```python
from build123d import *

# Parameters (mm, degrees)
BOSS_EXTRUDE1_DEPTH                 = 12.5
CUT_EXTRUDE1_REACH                  = 42.463
CUT_EXTRUDE1_END_RADIUS             = 9.5
CUT_EXTRUDE1_DIRECTION_2_REACH      = 42.463
CUT_EXTRUDE1_DIRECTION_2_END_RADIUS = 9.5
BOSS_EXTRUDE3_DEPTH                 = 6.35
SKETCH5_R                           = 2.5
BOSS_EXTRUDE4_DEPTH                 = 6.35
BOSS_EXTRUDE5_START                 = -46
BOSS_EXTRUDE5_DEPTH                 = 46
BOSS_EXTRUDE6_DEPTH                 = 6.35
BOSS_EXTRUDE6_DRAFT                 = 10
HOLE1_START                         = 6.15
HOLE1_OUTLINE_R                     = 2.5
HOLE1_DEPTH                         = 52.35
FILLET1_R                           = 2.5


# Read off the part's stored shape, not the designer's step: Hole1
with BuildPart() as part:
    # Sketch1 → Boss-Extrude1 (new, symmetric)
    with BuildSketch(Plane.XY):
        with BuildLine():
            ThreePointArc((-9.5, 12.87439319), (-35, 0), (-9.5, -12.87439319))
            ThreePointArc((-9.5, -12.87439319), (0, -9.748786379), (9.5, -12.87439319))
            ThreePointArc((9.5, -12.87439319), (35, 0), (9.5, 12.87439319))
            ThreePointArc((9.5, 12.87439319), (0, 9.748786379), (-9.5, 12.87439319))
        make_face()
    extrude(amount=BOSS_EXTRUDE1_DEPTH, both=True)

    # Sketch2 → Cut-Revolve1 (revolve, cut)
    with BuildSketch(Plane(origin=(19, 0, 0), x_dir=(0, 0, -1), z_dir=(1, 0, 0)), mode=Mode.PRIVATE) as cut_revolve1_sk:
        Polygon((-12.5, 0), (-12.5, 14.25), (-6.5, 14.25), (-6.5, 12.5), (-4.5, 12.5), (-4.5, 11.5), (-2.5, 11.5), (-2.5, 9.5), (9.5, 9.5), (9.5, 4.5), (8.5, 4.5), (8.5, 0), align=None)
    cut_revolve1 = revolve(cut_revolve1_sk.sketch.rotate(Axis((19, 0, 0), (0, 0, 1)), 90), axis=Axis((19, 0, 0), (0, 0, 1)), mode=Mode.SUBTRACT)

    # Mirror1: Cut-Revolve1 across plane
    add(cut_revolve1.mirror(Plane(origin=(0, 0, 0), x_dir=(0, 0, 1), z_dir=(1, 0, 0))), mode=Mode.SUBTRACT)

    # Cut-Extrude1: up to this cylinder (the profile starts outside it)
    cut_extrude1_end = Plane(origin=(-19, 0, 0), z_dir=(0, 0, -1)) * Cylinder(CUT_EXTRUDE1_END_RADIUS, 104.926, mode=Mode.PRIVATE)
    # Sketch3 → Cut-Extrude1 (cut, up to the surface)
    with BuildSketch(Plane(origin=(0, 0, 0), x_dir=(0, 0, -1), z_dir=(1, 0, 0)), mode=Mode.PRIVATE) as cut_extrude1_sk1:
        with BuildLine():
            Line((0.75, -7.75), (-0.75, -7.75))
            ThreePointArc((-0.75, -7.75), (-1.810660172, -7.310660172), (-2.25, -6.25))
            Line((-2.25, -6.25), (-2.25, 6.25))
            ThreePointArc((-2.25, 6.25), (-1.810660172, 7.310660172), (-0.75, 7.75))
            Line((-0.75, 7.75), (0.75, 7.75))
            ThreePointArc((0.75, 7.75), (1.810660172, 7.310660172), (2.25, 6.25))
            Line((2.25, 6.25), (2.25, -6.25))
            ThreePointArc((2.25, -6.25), (1.810660172, -7.310660172), (0.75, -7.75))
        make_face()
    cut_extrude1_tool1 = extrude(cut_extrude1_sk1.sketch, amount=-CUT_EXTRUDE1_REACH, mode=Mode.PRIVATE) - cut_extrude1_end
    add(cut_extrude1_tool1.solids().sort_by_distance((0, 0, 0))[0], mode=Mode.SUBTRACT)

    # Cut-Extrude1 direction 2: up to this cylinder (the profile starts outside it)
    cut_extrude1_direction_2_end = Plane(origin=(19, 0, 0), z_dir=(0, 0, -1)) * Cylinder(CUT_EXTRUDE1_DIRECTION_2_END_RADIUS, 104.926, mode=Mode.PRIVATE)
    # Sketch3 → Cut-Extrude1 direction 2 (cut, up to the surface)
    with BuildSketch(Plane(origin=(0, 0, 0), x_dir=(0, 0, -1), z_dir=(1, 0, 0)), mode=Mode.PRIVATE) as cut_extrude1_direction_2_sk1:
        with BuildLine():
            Line((0.75, -7.75), (-0.75, -7.75))
            ThreePointArc((-0.75, -7.75), (-1.810660172, -7.310660172), (-2.25, -6.25))
            Line((-2.25, -6.25), (-2.25, 6.25))
            ThreePointArc((-2.25, 6.25), (-1.810660172, 7.310660172), (-0.75, 7.75))
            Line((-0.75, 7.75), (0.75, 7.75))
            ThreePointArc((0.75, 7.75), (1.810660172, 7.310660172), (2.25, 6.25))
            Line((2.25, 6.25), (2.25, -6.25))
            ThreePointArc((2.25, -6.25), (1.810660172, -7.310660172), (0.75, -7.75))
        make_face()
    cut_extrude1_direction_2_tool1 = extrude(cut_extrude1_direction_2_sk1.sketch, amount=CUT_EXTRUDE1_DIRECTION_2_REACH, mode=Mode.PRIVATE) - cut_extrude1_direction_2_end
    add(cut_extrude1_direction_2_tool1.solids().sort_by_distance((0, 0, 0))[0], mode=Mode.SUBTRACT)

    # Sketch4 → Boss-Extrude3 (add)
    with BuildSketch(Plane.XY.offset(12.5)):
        with BuildLine():
            Line((-45.380476721, -5.413087491), (-34.979470203, -0.810266645))
            ThreePointArc((-34.979470203, -0.810266645), (-31.820655502, -9.572397426), (-24.317188777, -15.090642912))
            Line((-24.317188777, -15.090642912), (-44.730811053, -13.974760557))
            ThreePointArc((-44.730811053, -13.974760557), (-47.485667167, -9.87831587), (-45.380476721, -5.413087491))
        make_face()
    boss_extrude3 = extrude(amount=-BOSS_EXTRUDE3_DEPTH)

    # Mirror2: Boss-Extrude3 across plane
    add(boss_extrude3.mirror(Plane(origin=(0, 0, 0), x_dir=(0, 0, 1), z_dir=(1, 0, 0))))

    # Sketch5 → Boss-Extrude4 (add)
    with BuildSketch(Plane.XY.offset(12.5)):
        with BuildLine():
            ThreePointArc((-14.279554898, 31.478453226), (-19, 34.83), (-23.720445102, 31.478453226))
            Line((-23.720445102, 31.478453226), (-31.028962191, 10.550074342))
            ThreePointArc((-31.028962191, 10.550074342), (-20.717418693, 15.907560248), (-9.5, 12.87439319))
            ThreePointArc((-9.5, 12.87439319), (-8.431487389, 12.150623988), (-7.308118696, 11.515325762))
            Line((-7.308118696, 11.515325762), (-14.279554898, 31.478453226))
        make_face()
        with Locations((-19, 29.83)):
            Circle(SKETCH5_R, mode=Mode.SUBTRACT)
    extrude(amount=-BOSS_EXTRUDE4_DEPTH)

    # Sketch6 → Boss-Extrude5 (add)
    with BuildSketch(Plane(origin=(0, 0, 6.15), x_dir=(-1, 0, 0), z_dir=(0, 0, -1)).offset(BOSS_EXTRUDE5_START)):
        with BuildLine():
            Line((44.730811053, -13.974760557), (24.317188777, -15.090642912))
            ThreePointArc((24.317188777, -15.090642912), (16.633162841, -15.823971747), (9.5, -12.87439319))
            ThreePointArc((9.5, -12.87439319), (0, -9.748786379), (-9.5, -12.87439319))
            ThreePointArc((-9.5, -12.87439319), (-16.633162841, -15.823971747), (-24.317188777, -15.090642912))
            Line((-24.317188777, -15.090642912), (-44.730811053, -13.974760557))
            ThreePointArc((-44.730811053, -13.974760557), (0, -32.403655151), (44.730811053, -13.974760557))
        make_face()
    extrude(amount=BOSS_EXTRUDE5_DEPTH)


with BuildPart() as boss_extrude6_tool:
    # Sketch7 → Boss-Extrude6 (with draft: the straight prism first)
    with BuildSketch(Plane.XY.offset(52.15)):
        with BuildLine():
            Line((-7.5, 15.5), (-7.5, 9.15))
            ThreePointArc((-7.5, 9.15), (-19, -2.35), (-30.5, 9.15))
            Line((-30.5, 9.15), (-30.5, 15.5))
            Line((-30.5, 15.5), (-40, 15.5))
            Line((-40, 15.5), (-40, 8.234972412))
            ThreePointArc((-40, 8.234972412), (-41.393677612, 0.899799121), (-45.380476721, -5.413087491))
            ThreePointArc((-45.380476721, -5.413087491), (-47.485667167, -9.87831587), (-44.730811053, -13.974760557))
            ThreePointArc((-44.730811053, -13.974760557), (0, -32.403655151), (44.730811053, -13.974760557))
            ThreePointArc((44.730811053, -13.974760557), (47.485667167, -9.87831587), (45.380476721, -5.413087491))
            ThreePointArc((45.380476721, -5.413087491), (41.393677612, 0.899799121), (40, 8.234972412))
            Line((40, 8.234972412), (40, 15.5))
            Line((40, 15.5), (30.5, 15.5))
            Line((30.5, 15.5), (30.5, 9.15))
            ThreePointArc((30.5, 9.15), (19, -2.35), (7.5, 9.15))
            Line((7.5, 9.15), (7.5, 15.5))
            Line((7.5, 15.5), (-7.5, 15.5))
        make_face()
    extrude(amount=BOSS_EXTRUDE6_DEPTH)
    # Boss-Extrude6: the draft: its side faces are tilted about the plane it starts from
    boss_extrude6_sides = [boss_extrude6_tool.faces().sort_by_distance(p)[0] for p in [
        (0, -32.403655151, 55.325),
        (47.485667167, -9.87831587, 55.325),
        (41.393677612, 0.899799121, 55.325),
        (40, 11.867486206, 55.325),
        (35.25, 15.5, 55.325),
        (30.5, 12.325, 55.325),
        (19, -2.35, 55.325),
        (7.5, 12.325, 55.325),
        (0, 15.5, 55.325),
        (-7.5, 12.325, 55.325),
        (-19, -2.35, 55.325),
        (-30.5, 12.325, 55.325),
        (-35.25, 15.5, 55.325),
        (-40, 11.867486206, 55.325),
        (-41.393677612, 0.899799121, 55.325),
        (-47.485667167, -9.87831587, 55.325),
    ]]
    draft(boss_extrude6_sides, Plane.XY.offset(52.15), BOSS_EXTRUDE6_DRAFT)


with BuildPart() as part_1:
    add(part.part)

    # Boss-Extrude6: add boss_extrude6_tool
    add(boss_extrude6_tool.part)

    # Hole1 outline → Hole1 (cut)
    with BuildSketch(Plane.XY.offset(HOLE1_START)):
        with Locations((42.5, -9.5)):
            Circle(HOLE1_OUTLINE_R)
    hole1 = extrude(amount=HOLE1_DEPTH, mode=Mode.SUBTRACT)

    # Mirror3: Hole1 across plane
    add(hole1.mirror(Plane(origin=(0, 0, 0), x_dir=(0, 0, 1), z_dir=(1, 0, 0))), mode=Mode.SUBTRACT)

    # Fillet1
    fillet1_edges = [part_1.edges().sort_by_distance(p)[0] for p in [
        (35, 0, -12.5),
        (0, -9.748786379, -12.5),
        (-35, 0, -12.5),
        (0, 9.748786379, -12.5),
    ]]
    fillet(fillet1_edges, radius=FILLET1_R)


solid = part_1.part
```
Work out the finished part from the listing and answer in its coordinate system (mm). A direction names the side the tool comes from. Coordinates: 2 decimals unless noted, no trailing zeros. Loops run counter-clockwise (first coordinate to the right, second up) from the corner with the lowest first, then second, coordinate; pieces in that order, holes last. Notation, with made-up numbers: (89, 89.25) - (143, 89.25) arc R12 ccw to (143, 102.25) - close; hole circle Ø1 at (0.25, -22). An arc over 180 degrees is marked (long way). Use a Markdown table: item, result.
Item 1: Consider probe 1 along X at (y, z) = (0, -5.75); probe 2 along Z at (x, y) = (-5, 1.5); probe 3 along Y at (x, z) = (-19.5, -9). Determine where each line is inside the solid, lowest interval first. Write a range as from..to.
Evaluation:
| item | result |
|---|---|
| probe 1 | x = -35..-28.5, -9.5..9.5, 28.5..35 |
| probe 2 | z = -12.5..-2.25, 2.25..6.5, 52.15..58.5 |
| probe 3 | y = -15.99..-9.49, -4.47..4.47, 9.49..15.99 |
Item 2: For faces 1 (the flat face through (-19, 0, -8.5)), 2 (the flat face through (-40.253, -3.144, 9.369)), 3 (the flat face through (34.38, -14.54, 32.6)), determine the directions among +Z, -Z, +X, -X, +Y, -Y from which every point of the face is accessible in a straight line to the end or side of a thin tool.
Evaluation:
| item | result |
|---|---|
| face 1 | none |
| face 2 | -Z, -X, +Y |
| face 3 | +Y |
Item 3: Find section B-B, the plane z = 31. Determine the outline of the cut face in (x, y).
Evaluation:
| item | result |
|---|---|
| outline | (-44.73, -13.97) arc R63.5 ccw to (44.73, -13.97) - (24.32, -15.09) arc R16 cw to (9.5, -12.87) arc R16 ccw to (-9.5, -12.87) arc R16 cw to (-24.32, -15.09) - close |
Item 4: Given pin 1 Ø6 at (x, z) = (-21.5, 27) entering from -Y; pin 2 Ø2.5 at (x, y) = (-17.5, 0) entering from +Z; pin 3 Ø2 at (y, z) = (-3, 3.5) entering from -X, each flat-ended and moving along its own axis, determine where each tip first touches the part or whether it passes through.
Evaluation:
| item | result |
|---|---|
| pin 1 | stops at y = -29.65 |
| pin 2 | stops at z = -8.5 |
| pin 3 | stops at x = -34.87 |
Item 5: Find section A-A, the plane y = 29.83. Determine the outline of the cut face in (x, z), and give its area (3 significant figures).
Evaluation:
| item | result |
|---|---|
| outline | (-24.3, 6.15) - (-21.5, 6.15) - (-21.5, 12.5) - (-24.3, 12.5) - close; (-16.5, 6.15) - (-13.7, 6.15) - (-13.7, 12.5) - (-16.5, 12.5) - close |
| area | 35.5 mm2 |
Item 6: Find section C-C, the plane x = 42.5. State how many separate pieces and enclosed holes the cut face has, and give its area (3 significant figures).
Evaluation:
| item | result |
|---|---|
| separate pieces | 3 |
| enclosed holes | 0 |
| area | 172 mm2 |
Item 7: The mould has two halves that part along Z. Classify faces 4 (the cylindrical face through (-8.03, -3.45, 3.49)), 5 (the cylindrical face through (44.81, -10.46, 55.28)), 6 (the flat face through (35.32, 14.95, 55.28)): +Z half, -Z half, draft (parallel to the pull), parting line (faces both ways), or undercut.
Evaluation:
| item | result |
|---|---|
| face 4 | undercut |
| face 5 | draft |
| face 6 | +Z half |
